```python
from build123d import *

# Parameters (mm, degrees)
SKETCH1_W               = 90
SKETCH1_H               = 120
BOSS_EXTRUDE1_DEPTH     = 2.5
CUT_EXTRUDE2_DEPTH      = 10
SKETCH4_W               = 90
SKETCH4_H               = 120
SKETCH4_W_2             = 86.4
SKETCH4_H_2             = 116.4
CUT_EXTRUDE4_DEPTH      = 1
FILLET2_R               = 4
FILLET3_R               = 4.512
CUT_EXTRUDE6_DEPTH      = 1.5
SKETCH5_R               = 1
CUT_EXTRUDE9_DEPTH      = 1.5
SKETCH6_R               = 1
CUT_EXTRUDE10_DEPTH     = 5
SKETCH7_R               = 1
CUT_EXTRUDE11_DEPTH     = 5
SKETCH8_R               = 1
CUT_EXTRUDE12_DEPTH     = 5
SKETCH9_R               = 1
CUT_EXTRUDE13_DEPTH     = 5
SKETCH10_R              = 1
CUT_EXTRUDE14_DEPTH     = 5
SKETCH11_R              = 1
CUT_EXTRUDE15_DEPTH     = 5
SKETCH12_R              = 1
CUT_EXTRUDE16_DEPTH     = 5
SKETCH13_R              = 1
CUT_EXTRUDE17_DEPTH     = 5
SKE_VAT_R               = 8
VAT_DEPTH               = 1
MIRROR3_COPY_1_SKETCH_R = 8
MIRROR3_COPY_1_DEPTH    = 1
MIRROR3_COPY_2_SKETCH_R = 8
MIRROR3_COPY_2_DEPTH    = 1
SKETCH18_W              = 10
SKETCH18_H              = 13
CUT_EXTRUDE19_DEPTH     = 1.5
SKETCH19_R              = 1.4
CUT_EXTRUDE20_DEPTH     = 10
MIRROR5_COPY_1_SKETCH_R = 1.4
MIRROR5_COPY_1_DEPTH    = 10


with BuildPart() as part:
    # Sketch1 → Boss-Extrude1 (new body)
    with BuildSketch(Plane.XY):
        Rectangle(SKETCH1_W, SKETCH1_H)
    extrude(amount=BOSS_EXTRUDE1_DEPTH)

    # Sketch2 → Cut-Extrude2 (cut)
    with BuildSketch(Plane.XY.offset(2.5)):
        Polygon((-30.25, -50.5), (0, -50.5), (30, -50.5), (30.5, -50.5), (30.5, 8.5), (-30.5, 8.5), (-30.5, -50.5), align=None)
        Polygon((0, 55.5), (23.75, 55.5), (23.75, 19.5), (-23.75, 19.5), (-23.75, 55.5), align=None)
    extrude(amount=-CUT_EXTRUDE2_DEPTH, mode=Mode.SUBTRACT)

    # Sketch4 → Cut-Extrude4 (cut)
    with BuildSketch(Plane(origin=(0, 0, 0), x_dir=(-1, 0, 0), z_dir=(0, 0, -1))):
        Rectangle(SKETCH4_W, SKETCH4_H)
        Rectangle(SKETCH4_W_2, SKETCH4_H_2, mode=Mode.SUBTRACT)
    extrude(amount=-CUT_EXTRUDE4_DEPTH, mode=Mode.SUBTRACT)

    # Fillet2
    fillet2_edges = [part.edges().sort_by_distance(p)[0] for p in [
        (-43.2, -58.2, 0.5),
        (43.2, -58.2, 0.5),
        (43.2, 58.2, 0.5),
        (-43.2, 58.2, 0.5),
        (45, -60, 1.75),
        (-45, -60, 1.75),
        (-45, 60, 1.75),
        (45, 60, 1.75),
    ]]
    fillet(fillet2_edges, radius=FILLET2_R)

    # Fillet3
    fillet3_edges = [part.edges().sort_by_distance(p)[0] for p in [
        (-30.5, -50.5, 1.25),
        (-30.5, 8.5, 1.25),
        (30.5, 8.5, 1.25),
        (30.5, -50.5, 1.25),
    ]]
    fillet(fillet3_edges, radius=FILLET3_R)

    # Sketch2_4 → Cut-Extrude6 (cut)
    with BuildSketch(Plane.XY.offset(2.5)):
        with BuildLine():
            ThreePointArc((-25.7, 52.2), (-24.992893219, 52.492893219), (-24.7, 53.2))
            Line((-24.7, 53.2), (-25.7, 53.2))
            Line((-25.7, 53.2), (-25.7, 52.2))
        make_face()
        with BuildLine():
            Line((-25.7, 53.2), (-24.7, 53.2))
            ThreePointArc((-24.7, 53.2), (-26.407106781, 53.907106781), (-25.7, 52.2))
            Line((-25.7, 52.2), (-25.7, 53.2))
        make_face()
        with BuildLine():
            ThreePointArc((-24.7, 21.8), (-24.992893219, 22.507106781), (-25.7, 22.8))
            Line((-25.7, 22.8), (-25.7, 21.8))
            Line((-25.7, 21.8), (-24.7, 21.8))
        make_face()
        with BuildLine():
            Line((-25.7, 21.8), (-25.7, 22.8))
            ThreePointArc((-25.7, 22.8), (-26.407106781, 21.092893219), (-24.7, 21.8))
            Line((-24.7, 21.8), (-25.7, 21.8))
        make_face()
        with BuildLine():
            ThreePointArc((25.7, 22.8), (24.992893219, 22.507106781), (24.7, 21.8))
            Line((24.7, 21.8), (25.7, 21.8))
            Line((25.7, 21.8), (25.7, 22.8))
        make_face()
        with BuildLine():
            Line((25.7, 21.8), (24.7, 21.8))
            ThreePointArc((24.7, 21.8), (25.7, 20.8), (26.7, 21.8))
            ThreePointArc((26.7, 21.8), (26.407106781, 22.507106781), (25.7, 22.8))
            Line((25.7, 22.8), (25.7, 21.8))
        make_face()
        with BuildLine():
            ThreePointArc((26.7, 53.2), (25.7, 54.2), (24.7, 53.2))
            Line((24.7, 53.2), (25.7, 53.2))
            Line((25.7, 53.2), (25.7, 52.2))
            ThreePointArc((25.7, 52.2), (26.407106781, 52.492893219), (26.7, 53.2))
        make_face()
        with BuildLine():
            Line((25.7, 53.2), (24.7, 53.2))
            ThreePointArc((24.7, 53.2), (24.992893219, 52.492893219), (25.7, 52.2))
            Line((25.7, 52.2), (25.7, 53.2))
        make_face()
    extrude(amount=-CUT_EXTRUDE6_DEPTH, mode=Mode.SUBTRACT)

    # Sketch5 → Cut-Extrude9 (cut)
    with BuildSketch(Plane.XY.offset(2.5)):
        with Locations((-30, 8.5)):
            Circle(SKETCH5_R)
        with Locations((-30, -50.5)):
            Circle(SKETCH5_R)
        with Locations((30, 8.5)):
            Circle(SKETCH5_R)
        with Locations((30, -50.5)):
            Circle(SKETCH5_R)
    extrude(amount=-CUT_EXTRUDE9_DEPTH, mode=Mode.SUBTRACT)

    # Sketch6 → Cut-Extrude10 (cut)
    with BuildSketch(Plane.XY.offset(2.5)):
        with Locations((-30, 8.5)):
            Circle(SKETCH6_R)
    extrude(amount=-CUT_EXTRUDE10_DEPTH, mode=Mode.SUBTRACT)

    # Sketch7 → Cut-Extrude11 (cut)
    with BuildSketch(Plane.XY.offset(2.5)):
        with Locations((30, 8.5)):
            Circle(SKETCH7_R)
    extrude(amount=-CUT_EXTRUDE11_DEPTH, mode=Mode.SUBTRACT)

    # Sketch8 → Cut-Extrude12 (cut)
    with BuildSketch(Plane.XY.offset(2.5)):
        with Locations((-25.7, 21.8)):
            Circle(SKETCH8_R)
    extrude(amount=-CUT_EXTRUDE12_DEPTH, mode=Mode.SUBTRACT)

    # Sketch9 → Cut-Extrude13 (cut)
    with BuildSketch(Plane.XY.offset(2.5)):
        with Locations((25.7, 21.8)):
            Circle(SKETCH9_R)
    extrude(amount=-CUT_EXTRUDE13_DEPTH, mode=Mode.SUBTRACT)

    # Sketch10 → Cut-Extrude14 (cut)
    with BuildSketch(Plane.XY.offset(2.5)):
        with Locations((-30, -50.5)):
            Circle(SKETCH10_R)
    extrude(amount=-CUT_EXTRUDE14_DEPTH, mode=Mode.SUBTRACT)

    # Sketch11 → Cut-Extrude15 (cut)
    with BuildSketch(Plane.XY.offset(2.5)):
        with Locations((30, -50.5)):
            Circle(SKETCH11_R)
    extrude(amount=-CUT_EXTRUDE15_DEPTH, mode=Mode.SUBTRACT)

    # Sketch12 → Cut-Extrude16 (cut)
    with BuildSketch(Plane.XY.offset(2.5)):
        with Locations((25.7, 53.2)):
            Circle(SKETCH12_R)
    extrude(amount=-CUT_EXTRUDE16_DEPTH, mode=Mode.SUBTRACT)

    # Sketch13 → Cut-Extrude17 (cut)
    with BuildSketch(Plane.XY.offset(2.5)):
        with Locations((-25.7, 53.2)):
            Circle(SKETCH13_R)
    extrude(amount=-CUT_EXTRUDE17_DEPTH, mode=Mode.SUBTRACT)

    # ske_vat → vat (cut)
    with BuildSketch(Plane(origin=(0, 0, 0), x_dir=(1, 0, 0), z_dir=(0, 0, -1))):
        with Locations((42.028427125, -57.028427125)):
            Circle(SKE_VAT_R)
    vat = extrude(amount=-VAT_DEPTH, mode=Mode.SUBTRACT)

    # Mirror1: vat across plane
    add(vat.mirror(Plane(origin=(0, 0, 0), x_dir=(0, 0, 1), z_dir=(1, 0, 0))), mode=Mode.SUBTRACT)

    # Mirror2: vat across plane
    add(vat.mirror(Plane.ZX), mode=Mode.SUBTRACT)

    # Mirror3 copy 1 sketch → Mirror3 copy 1 (cut)
    with BuildSketch(Plane(origin=(0, 0, 0), x_dir=(-1, 0, 0), z_dir=(0, 0, -1))):
        with Locations((42.028427125, -57.028427125)):
            Circle(MIRROR3_COPY_1_SKETCH_R)
    extrude(amount=-MIRROR3_COPY_1_DEPTH, mode=Mode.SUBTRACT)

    # Mirror3 copy 2 sketch → Mirror3 copy 2 (cut)
    with BuildSketch(Plane(origin=(0, 0, 0), x_dir=(-1, 0, 0), z_dir=(0, 0, -1))):
        with Locations((42.028427125, 57.028427125)):
            Circle(MIRROR3_COPY_2_SKETCH_R)
    extrude(amount=-MIRROR3_COPY_2_DEPTH, mode=Mode.SUBTRACT)

    # Sketch18 → Cut-Extrude19 (cut)
    with BuildSketch(Plane(origin=(0, 0, 0), x_dir=(1, 0, 0), z_dir=(0, 0, -1))):
        with Locations((-28.75, -31)):
            Rectangle(SKETCH18_W, SKETCH18_H)
        with Locations((-28.75, -44)):
            Rectangle(SKETCH18_W, SKETCH18_H)
    extrude(amount=-CUT_EXTRUDE19_DEPTH, mode=Mode.SUBTRACT)

    # Sketch19 → Cut-Extrude20 (cut)
    with BuildSketch(Plane(origin=(0, 0, 1), x_dir=(1, 0, 0), z_dir=(0, 0, -1))):
        with Locations(Location((39.939339828, -54.939339828, 0), (0, 0, 180))):
            Circle(SKETCH19_R)
    cut_extrude20 = extrude(amount=-CUT_EXTRUDE20_DEPTH, mode=Mode.SUBTRACT)

    # Mirror4: Cut-Extrude20 across plane
    add(cut_extrude20.mirror(Plane(origin=(0, 0, 0), x_dir=(0, 0, 1), z_dir=(1, 0, 0))), mode=Mode.SUBTRACT)

    # Mirror5: Cut-Extrude20 across plane
    add(cut_extrude20.mirror(Plane.ZX), mode=Mode.SUBTRACT)

    # Mirror5 copy 1 sketch → Mirror5 copy 1 (cut)
    with BuildSketch(Plane(origin=(0, 0, 1), x_dir=(-1, 0, 0), z_dir=(0, 0, -1))):
        with Locations(Location((39.939339828, -54.939339828, 0), (0, 0, 180))):
            Circle(MIRROR5_COPY_1_SKETCH_R)
    extrude(amount=-MIRROR5_COPY_1_DEPTH, mode=Mode.SUBTRACT)


solid = part.part
```
Part model, mm, in its own coordinate system. A direction names the side the tool comes from. Give positions to 0.01 mm unless a question says otherwise; leave off trailing zeros. Order: outer loops, then holes, each group sorted by start corner. A loop starts at its lowest first (then second) coordinate and runs counter-clockwise, first axis right, second up. Notation, with made-up numbers: M 80,41 L 112,41 A19 ccw 112,75 Z; hole C -4,-31.75 d10. An arc over 180 degrees is marked long. Use a Markdown table: item, result. Add a question column.
(1) Drop flat-ended pins along their axis: P1, Ø0.8, axis at y = 16.5, z = 0.5, coming from the -X side; P2, Ø0.5, axis at x = -13.5, z = 0.5, coming from the +Y side. Give the stop position or say it passes through.
(2) 3-axis set-ups, long thin cutter, end or side, ignore diameter. For faces 5 (the face through (-29, 37, 1.5)), 6 (the face through (0, 19.5, 1)): which of +Z, -Z, +X, -X, +Y, -Y reach the whole face in a straight line?
(3) Saw through at C-C, the plane z = 0.4. Give the number of separate pieces and of enclosed holes in the cut face, and give its area (3 significant figures).
(4) Saw through at A-A, the plane x = 3. Give the cut face in (y, z), and give its area (3 significant figures).
(5) Saw through at D-D, the plane y = 37. Give the cut face in (x, z).
(6) Probe line 1 along Y through (x, z) = (10, 2.4); line 2 along Y through (x, z) = (25.7, 1.45); line 3 along X through (y, z) = (4, 2.25). List the from-to ranges inside material, lowest first. Write a range as [from, to].
(7) Saw through at B-B, the plane y = -15.5. Give the cut face in (x, z).
(8) Mould opens along Y. For faces 1 (the face through (-1, 14, 0)), 2 (the face through (-43.859, -58.797, 1.76)), 3 (the face through (0, 55.5, 1)), 4 (the face through (43.797, 58.859, 1.76)) say: +Y half, -Y half, draft (parallel to the pull), parting line (faces both ways), or undercut.
Answer key:
| question | item | result |
|---|---|---|
| 1 | P1 | x = -43.2 |
| 1 | P2 | y = 58.2 |
| 2 | face 5 | -Z |
| 2 | face 6 | +Z, -Z |
| 3 | separate pieces | 1 |
| 3 | enclosed holes | 10 |
| 3 | area | 4,200 mm^2 |
| 4 | outline | M -60,1 L -58.2,1 L -58.2,0 L -50.5,0 L -50.5,2.5 L -60,2.5 Z; M 8.5,0 L 19.5,0 L 19.5,2.5 L 8.5,2.5 Z; M 55.5,0 L 58.2,0 L 58.2,1 L 60,1 L 60,2.5 L 55.5,2.5 Z |
| 4 | area | 58.9 mm^2 |
| 5 | outline | M -45,1 L -43.2,1 L -43.2,0 L -33.75,0 L -33.75,1.5 L -23.75,1.5 L -23.75,2.5 L -45,2.5 Z; M 23.75,0 L 43.2,0 L 43.2,1 L 45,1 L 45,2.5 L 23.75,2.5 Z |
| 6 | line 1 | [-60, -50.5], [8.5, 19.5], [55.5, 60] |
| 6 | line 2 | [-60, -50.5], [8.5, 20.8], [22.8, 52.2], [54.2, 60] |
| 6 | line 3 | [-45, -30.5], [30.5, 45] |
| 7 | outline | M -45,1 L -43.2,1 L -43.2,0 L -30.5,0 L -30.5,2.5 L -45,2.5 Z; M 30.5,0 L 43.2,0 L 43.2,1 L 45,1 L 45,2.5 L 30.5,2.5 Z |
| 8 | face 1 | draft |
| 8 | face 2 | -Y half |
| 8 | face 3 | undercut |
| 8 | face 4 | +Y half |
